```python
from build123d import *

# Parameters (mm, degrees)
F0_R     = 16
F0_R_2   = 1.5
F0_R_3   = 2.5
F1_DEPTH = 62


with BuildPart() as f1:
    # F0 (on Top) → F1 (new body)
    with BuildSketch(Plane.XY):
        Circle(F0_R)
        with Locations((-10.401443, -9.813255)):
            Circle(F0_R_2, mode=Mode.SUBTRACT)
        with Locations((-4.890888, -13.437604)):
            Circle(F0_R_2, mode=Mode.SUBTRACT)
        with Locations((-1.660129, -14.203309)):
            Circle(F0_R_2, mode=Mode.SUBTRACT)
        with Locations((-7.857978, -11.947476)):
            Circle(F0_R_2, mode=Mode.SUBTRACT)
        with Locations((-6.465638, -8.899187)):
            Circle(F0_R_2, mode=Mode.SUBTRACT)
        with Locations((-3.399187, -10.461622)):
            Circle(F0_R_2, mode=Mode.SUBTRACT)
        with Locations((-12.384163, -7.15)):
            Circle(F0_R_2, mode=Mode.SUBTRACT)
        with Locations((-13.69925, -4.101286)):
            Circle(F0_R_2, mode=Mode.SUBTRACT)
        with Locations((-8.899187, -6.465638)):
            Circle(F0_R_2, mode=Mode.SUBTRACT)
        with Locations((-14.275807, -0.831471)):
            Circle(F0_R_2, mode=Mode.SUBTRACT)
        with Locations((-10.461622, -3.399187)):
            Circle(F0_R_2, mode=Mode.SUBTRACT)
        with Locations((-6.020102, -4.800871)):
            Circle(F0_R_2, mode=Mode.SUBTRACT)
        with Locations((-3.340905, -6.93746)):
            Circle(F0_R_2, mode=Mode.SUBTRACT)
        with Locations((-7.506945, -1.713411)):
            Circle(F0_R_2, mode=Mode.SUBTRACT)
        with Locations((-4.211534, -0.961255)):
            Circle(F0_R_2, mode=Mode.SUBTRACT)
        with Locations((-1.874309, -3.892043)):
            Circle(F0_R_2, mode=Mode.SUBTRACT)
        with Locations((1.660129, -14.203309)):
            Circle(F0_R_2, mode=Mode.SUBTRACT)
        with Locations((4.890888, -13.437604)):
            Circle(F0_R_2, mode=Mode.SUBTRACT)
        with Locations((0, -11)):
            Circle(F0_R_2, mode=Mode.SUBTRACT)
        with Locations((3.399187, -10.461622)):
            Circle(F0_R_2, mode=Mode.SUBTRACT)
        with Locations((7.857978, -11.947476)):
            Circle(F0_R_2, mode=Mode.SUBTRACT)
        with Locations((6.465638, -8.899187)):
            Circle(F0_R_2, mode=Mode.SUBTRACT)
        with Locations((10.401443, -9.813255)):
            Circle(F0_R_2, mode=Mode.SUBTRACT)
        with Locations((0, -7.7)):
            Circle(F0_R_2, mode=Mode.SUBTRACT)
        with Locations((3.340905, -6.93746)):
            Circle(F0_R_2, mode=Mode.SUBTRACT)
        with Locations((6.020102, -4.800871)):
            Circle(F0_R_2, mode=Mode.SUBTRACT)
        with Locations((1.874309, -3.892043)):
            Circle(F0_R_2, mode=Mode.SUBTRACT)
        with Locations((4.211534, -0.961255)):
            Circle(F0_R_2, mode=Mode.SUBTRACT)
        with Locations((7.506945, -1.713411)):
            Circle(F0_R_2, mode=Mode.SUBTRACT)
        with Locations((8.899187, -6.465638)):
            Circle(F0_R_2, mode=Mode.SUBTRACT)
        with Locations((12.384163, -7.15)):
            Circle(F0_R_2, mode=Mode.SUBTRACT)
        with Locations((13.69925, -4.101286)):
            Circle(F0_R_2, mode=Mode.SUBTRACT)
        with Locations((10.461622, -3.399187)):
            Circle(F0_R_2, mode=Mode.SUBTRACT)
        with Locations((14.275807, -0.831471)):
            Circle(F0_R_2, mode=Mode.SUBTRACT)
        with Locations((-14.082751, 2.483169)):
            Circle(F0_R_2, mode=Mode.SUBTRACT)
        with Locations((-11, 0)):
            Circle(F0_R_2, mode=Mode.SUBTRACT)
        with Locations((-10.461622, 3.399187)):
            Circle(F0_R_2, mode=Mode.SUBTRACT)
        with Locations((-13.13049, 5.663941)):
            Circle(F0_R_2, mode=Mode.SUBTRACT)
        with Locations((-8.899187, 6.465638)):
            Circle(F0_R_2, mode=Mode.SUBTRACT)
        with Locations((-7.506945, 1.713411)):
            Circle(F0_R_2, mode=Mode.SUBTRACT)
        with Locations((-3.377388, 2.693377)):
            Circle(F0_R_2, mode=Mode.SUBTRACT)
        with Locations((-6.020102, 4.800871)):
            Circle(F0_R_2, mode=Mode.SUBTRACT)
        with Locations((-3.340905, 6.93746)):
            Circle(F0_R_2, mode=Mode.SUBTRACT)
        with Locations((-11.470362, 8.539368)):
            Circle(F0_R_2, mode=Mode.SUBTRACT)
        with Locations((-9.191863, 10.954436)):
            Circle(F0_R_2, mode=Mode.SUBTRACT)
        with Locations((-6.465638, 8.899187)):
            Circle(F0_R_2, mode=Mode.SUBTRACT)
        with Locations((-3.399187, 10.461622)):
            Circle(F0_R_2, mode=Mode.SUBTRACT)
        with Locations((-6.417828, 12.778947)):
            Circle(F0_R_2, mode=Mode.SUBTRACT)
        with Locations((-3.297807, 13.914542)):
            Circle(F0_R_2, mode=Mode.SUBTRACT)
        Circle(F0_R_3, mode=Mode.SUBTRACT)
        with Locations((3.377388, 2.693377)):
            Circle(F0_R_2, mode=Mode.SUBTRACT)
        with Locations((7.506945, 1.713411)):
            Circle(F0_R_2, mode=Mode.SUBTRACT)
        with Locations((0, 4.319842)):
            Circle(F0_R_2, mode=Mode.SUBTRACT)
        with Locations((0, 7.7)):
            Circle(F0_R_2, mode=Mode.SUBTRACT)
        with Locations((3.340905, 6.93746)):
            Circle(F0_R_2, mode=Mode.SUBTRACT)
        with Locations((6.020102, 4.800871)):
            Circle(F0_R_2, mode=Mode.SUBTRACT)
        with Locations((11, 0)):
            Circle(F0_R_2, mode=Mode.SUBTRACT)
        with Locations((10.461622, 3.399187)):
            Circle(F0_R_2, mode=Mode.SUBTRACT)
        with Locations((14.082751, 2.483169)):
            Circle(F0_R_2, mode=Mode.SUBTRACT)
        with Locations((8.899187, 6.465638)):
            Circle(F0_R_2, mode=Mode.SUBTRACT)
        with Locations((13.13049, 5.663941)):
            Circle(F0_R_2, mode=Mode.SUBTRACT)
        with Locations((0, 11)):
            Circle(F0_R_2, mode=Mode.SUBTRACT)
        with Locations((3.399187, 10.461622)):
            Circle(F0_R_2, mode=Mode.SUBTRACT)
        with Locations((6.465638, 8.899187)):
            Circle(F0_R_2, mode=Mode.SUBTRACT)
        with Locations((3.297807, 13.914542)):
            Circle(F0_R_2, mode=Mode.SUBTRACT)
        with Locations((0, 14.3)):
            Circle(F0_R_2, mode=Mode.SUBTRACT)
        with Locations((6.417828, 12.778947)):
            Circle(F0_R_2, mode=Mode.SUBTRACT)
        with Locations((11.470362, 8.539368)):
            Circle(F0_R_2, mode=Mode.SUBTRACT)
        with Locations((9.191863, 10.954436)):
            Circle(F0_R_2, mode=Mode.SUBTRACT)
    extrude(amount=F1_DEPTH)


solid = f1.part
```
CAD build for the part. Positions are in the model's coordinates, mm. Round coordinates to 2 decimals unless told otherwise and drop trailing zeros. Use a Markdown table: item, result. Add a question column.
(1) Pull direction Y, two halves, no side cores. Call faces 1 (the face through (-4.59, -11.374, 30.566)), 2 (the face through (5.36, 9.91, 30.57)): +Y half, -Y half, draft (parallel to the pull), parting line (faces both ways), or undercut.
(2) Drill centre lines: line 1 (X direction, y = 10.5, z = 20); line 2 (X direction, y = 14, z = 40). Where is each one in solid material? Low to high.
(3) Cut at A-A (z = 36). State how many separate pieces and enclosed holes the cut face has, and give its area (3 significant figures).
(4) Flat gauge pins, fed straight in: pin 1 (5 mm diameter, centred on x = -6.5, z = 47, fed in from -Y); pin 2 (12 mm diameter, centred on x = 9, z = 16.5, fed in from -Y); pin 3 (1 mm diameter, centred on x = 3, z = 23.5, fed in from +Y). Where does each tip first touch, or does it go through?
Geometry says:
| question | item | result |
|---|---|---|
| 1 | face 1 | undercut |
| 1 | face 2 | undercut |
| 2 | line 1 | x = -12.07 to -10.62, -7.76 to -4.9, -1.9 to -1.41, 1.41 to 1.9, 4.9 to 7.76, 10.62 to 12.07 |
| 2 | line 2 | x = -7.75 to -7.29, -5.55 to -4.8, -1.8 to -1.47, 1.47 to 1.8, 4.8 to 5.55, 7.29 to 7.75 |
| 3 | separate pieces | 1 |
| 3 | enclosed holes | 69 |
| 3 | area | 304 mm² |
| 4 | pin 1 | stops at y = -15.49 |
| 4 | pin 2 | stops at y = -15.72 |
| 4 | pin 3 | stops at y = 15.8 |
